Geometry check sheet. Reference: the model listing, model coordinates, mm. Face numbers are marked on the shaded views. A direction names the side the tool comes from. Coordinates: 2 decimals unless noted, no trailing zeros. Write each loop counter-clockwise with the first axis right and the second up, starting at its lowest first coordinate (ties: lowest second). Pieces come first, ordered by that corner, then holes. Notation, with made-up numbers: (62.25, -8) -> (115.25, -8) arc R27 cw to (115.25, 11) -> close; hole circle Ø6 at (-33.5, -5). An arc over 180 degrees is marked (long way). One line per question, with ' | ' between items.
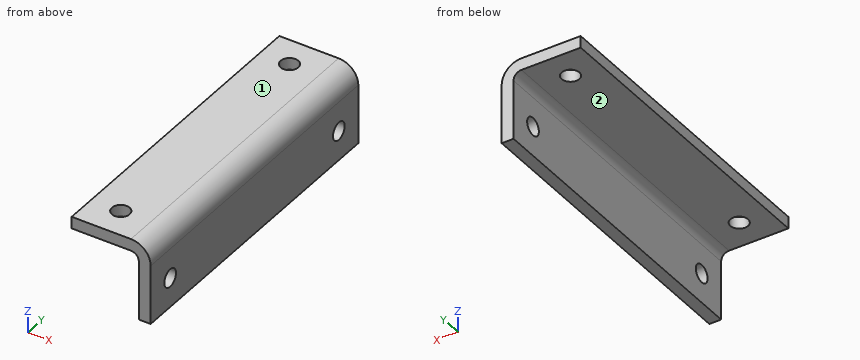
Autodesk Inventor part; units mm, degrees
ref_plane "YZ Plane" through (0, 0, 0) normal (1, 0, 0) x (0, 1, 0)
ref_plane "XZ Plane" through (0, 0, 0) normal (0, 1, 0) x (-1, 0, 0)
ref_plane "XY Plane" through (0, 0, 0) normal (0, 0, 1) x (1, 0, 0)
sketch "Sketch1" plane through (0, 0, 0) normal (0, 1, 0) x (-1, 0, 0)
  line L0 (0, 0) -> (20, 0)
  line L1 (20, 0) -> (20, -3)
  line L2 (20, -3) -> (0, -3)
  line L3 (0, -3) -> (0, 0)
  line L4 (0, 0) -> (3, 0)
  line L5 (3, 0) -> (3, -20)
  line L6 (3, -20) -> (0, -20)
  line L7 (0, -20) -> (0, 0)
  dimension "d0" = 3
  dimension "d1" = 3
  dimension "d2" = 20
  dimension "d3" = 20
extrude "Extrusion1" add sketch "Sketch1" along normal blind 80
fillet "Fillet1" radius 2 1 edges at (-3, 40, -3)
fillet "Fillet2" radius 5 1 edges at (0, 40, 0)
sketch "Sketch2" plane through (-3, 0, -20) normal (-1, 0, 0) x (0, 0, 1)
  line L0 (0, 80) -> (15, 80)
  line L1 (0, 0) -> (15, 0)
  line L2 (0, 0) -> (0, 80)
  point P0 (20, 0)
  point P1 (7.5, 72.5)
  point P2 (7.5, 7.5)
  dimension "d8" = 7.5
  dimension "d9" = 7.5
  dimension "d10" = 65
  dimension "d11" = 7.5
hole "Hole1" at (-3, 72.5, -12.5) at (-3, 7.5, -12.5) direction (1, 0, 0) diameter 4.5 end through all
sketch "Sketch3" plane through (-20, 0, -3) normal (0, 0, -1) x (-1, 0, 0)
  line L0 (-15, 80) -> (0, 80)
  line L1 (-15, 0) -> (0, 0)
  line L2 (0, 0) -> (0, 80)
  point P0 (-20, 0)
  point P1 (-7.5, 72.5)
  point P2 (-7.5, 7.5)
  dimension "d19" = 7.5
  dimension "d20" = 7.5
  dimension "d21" = 7.5
  dimension "d29" = 65
hole "Hole2" at (-12.5, 72.5, -3) at (-12.5, 7.5, -3) direction (0, 0, 1) diameter 4.5 end through all
equation "\"d1\" = d0"
equation "\"d3\" = d2"
properties part number "Timing_Angle Bracket" material "Aluminum 6061"
(1) Material ranges on line 1 (Y direction, x = -0.85, z = -12.5); line 2 (Z direction, x = -12.25, y = 45), recorded low to high.
Answers below:
line 1: y = 0 to 5.25, 9.75 to 70.25, 74.75 to 80 | line 2: z = -3 to 0
(2) Cross-section at C-C (z = -12.5). Record the cut outline in (x, y), plus the area to 3 significant figures.
Answers below:
outline: (-3, 0) -> (0, 0) -> (0, 5.25) -> (-3, 5.25) -> close; (-3, 9.75) -> (0, 9.75) -> (0, 70.25) -> (-3, 70.25) -> close; (-3, 74.75) -> (0, 74.75) -> (0, 80) -> (-3, 80) -> close | area: 213 mm²
(3) Cross-section at D-D (y = 65). Record the cut outline in (x, z), plus the area to 3 significant figures.
Answers below:
outline: (-20, -3) -> (-5, -3) arc R2 cw to (-3, -5) -> (-3, -20) -> (0, -20) -> (0, -5) arc R5 ccw to (-5, 0) -> (-20, 0) -> close | area: 106 mm²
(4) Cross-section at B-B (y = 7.5). Record the cut outline in (x, z).
Answers below:
outline: (-20, -3) -> (-14.75, -3) -> (-14.75, 0) -> (-20, 0) -> close; (-10.25, -3) -> (-5, -3) arc R2 cw to (-3, -5) -> (-3, -10.25) -> (0, -10.25) -> (0, -5) arc R5 ccw to (-5, 0) -> (-10.25, 0) -> close; (-3, -20) -> (0, -20) -> (0, -14.75) -> (-3, -14.75) -> close
(5) Cross-section at A-A (x = -12.5). Record the cut outline in (y, z).
Answers below:
outline: (0, -3) -> (5.25, -3) -> (5.25, 0) -> (0, 0) -> close; (9.75, -3) -> (70.25, -3) -> (70.25, 0) -> (9.75, 0) -> close; (74.75, -3) -> (80, -3) -> (80, 0) -> (74.75, 0) -> close
(6) Tool access check on the marked faces 1 and 2. Record the directions out of +Z, -Z, +X, -X, +Y, -Y that give a thin tool (end or side, any length) a straight path to the whole face; none if there is none.
Answers below:
face 1: +Z, +X, -X, +Y, -Y | face 2: -Z, -X, +Y, -Y
(7) Depth check by flat-ended pin: P1, Ø6, axis at y = 36.5, z = -15.5, coming from the -X side; P2, Ø6, axis at x = -9.5, y = 62.5, coming from the -Z side; P3, Ø5, axis at x = -7.5, z = -17.5, coming from the -Y side. Enter the tip coordinate at first touch or a pass-through.
Answers below:
P1: stops at x = -3 | P2: stops at z = -3 | P3: passes through
